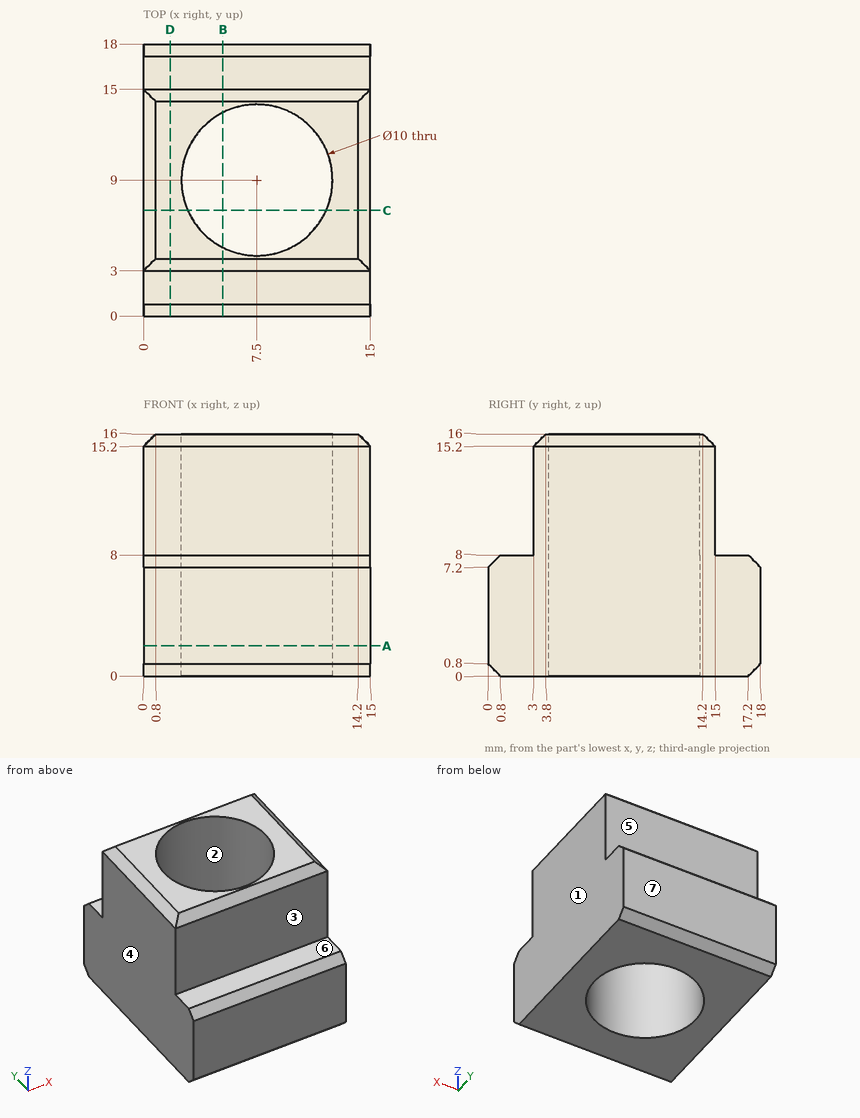
Study the drawing (mm; zero at the part's minimum x, y, z) and answer. A direction names the side the tool comes from. Give positions to 0.01 mm unless a question says otherwise; leave off trailing zeros. Loops run counter-clockwise (first coordinate to the right, second up) from the corner with the lowest first, then second, coordinate; pieces in that order, holes last. Notation, with made-up numbers: (-8.75, 74) -> (18.25, 74) arc R18 cw to (18.25, 100) -> close; hole circle Ø4 at (69.5, 75). An arc over 180 degrees is marked (long way). Use a Markdown table: item, result. Add a question column.
1) The part is cut by section B-B, the plane x = 5.25. Determine the outline of the cut face in (y, z).
2) The part is cut by section C-C, the plane y = 7. Determine the outline of the cut face in (x, z), plus the area to 3 significant figures.
3) The part is cut by section D-D, the plane x = 1.75. Determine the outline of the cut face in (y, z), plus the area to 3 significant figures.
4) The part is cut by section A-A, the plane z = 2. Determine the outline of the cut face in (x, y), plus the area to 3 significant figures.
5) Which of the six approach directions +Z, -Z, +X, -X, +Y, -Y give full straight-line access (tool end or side, diameter ignored) to the marked faces 5, 6 and 7?
6) Consider line 1 along X through (y, z) = (9, 7.5); line 2 along Z through (x, y) = (11, 1.75); line 3 along Y through (x, z) = (3.5, 12.5). Determine where each line is inside the solid, lowest interval first.
7) For a pull along X with two mould halves and no side action, classify the marked faces 1, 2, 3 and 4 as +X half, -X half, draft (parallel to the pull), parting line (faces both ways), or undercut.
8) Each of these flat-tipped pins is pushed along its axis until it touches: P1, Ø0.7, axis at x = 5.5, y = 2, coming from the +Z side; P2, Ø8, axis at x = 4.5, z = 13, coming from the +Y side. Where does it stop, or does it pass through?
Reported:
| question | item | result |
|---|---|---|
| 1 | outline | (0, 0.8) -> (0.8, 0) -> (4.53, 0) -> (4.53, 16) -> (3.8, 16) -> (3, 15.2) -> (3, 8) -> (0.8, 8) -> (0, 7.2) -> close; (13.47, 0) -> (17.2, 0) -> (18, 0.8) -> (18, 7.2) -> (17.2, 8) -> (15, 8) -> (15, 15.2) -> (14.2, 16) -> (13.47, 16) -> close |
| 2 | outline | (0, 0) -> (2.92, 0) -> (2.92, 16) -> (0.8, 16) -> (0, 15.2) -> close; (12.08, 0) -> (15, 0) -> (15, 15.2) -> (14.2, 16) -> (12.08, 16) -> close |
| 2 | area | 92.7 mm^2 |
| 3 | outline | (0, 0.8) -> (0.8, 0) -> (17.2, 0) -> (18, 0.8) -> (18, 7.2) -> (17.2, 8) -> (15, 8) -> (15, 15.2) -> (14.2, 16) -> (3.8, 16) -> (3, 15.2) -> (3, 8) -> (0.8, 8) -> (0, 7.2) -> close |
| 3 | area | 238 mm^2 |
| 4 | outline | (0, 0) -> (15, 0) -> (15, 18) -> (0, 18) -> close; hole circle Ø10 at (7.5, 9) |
| 4 | area | 191 mm^2 |
| 5 | face 5 | +Z, +X, -X, +Y |
| 5 | face 6 | +Z, +X, -X, -Y |
| 5 | face 7 | +Z, -Z, +X, -X, +Y |
| 6 | line 1 | x = 0 to 2.5, 12.5 to 15 |
| 6 | line 2 | z = 0 to 8 |
| 6 | line 3 | y = 3 to 6, 12 to 15 |
| 7 | face 1 | +X half |
| 7 | face 2 | undercut |
| 7 | face 3 | draft |
| 7 | face 4 | -X half |
| 8 | P1 | stops at z = 8 |
| 8 | P2 | stops at y = 15 |
